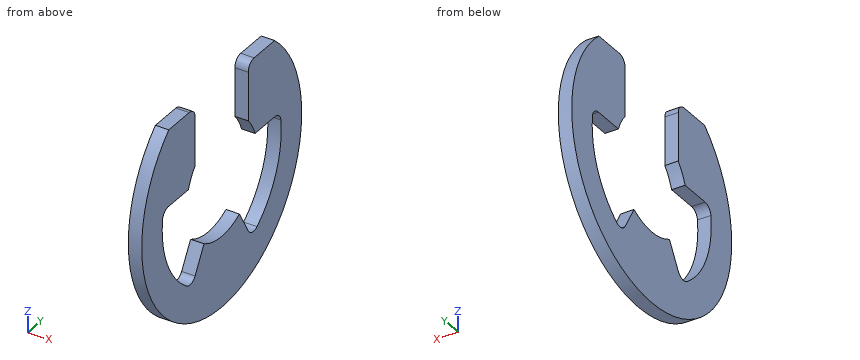
```python
from build123d import *

# Parameters (mm, degrees)
EXTRUDE1_DEPTH = 0.4445
FILLET1_R      = 0.6223


with BuildPart() as part:
    # Sketch1 → Extrude1 (new body, symmetric)
    with BuildSketch(Plane(origin=(0, 0, 0), x_dir=(0, 0, -1), z_dir=(1, 0, 0))):
        with BuildLine():
            Line((-2.45287604, 2.7813), (-6.2865, 2.7813))
            Line((-6.2865, 2.7813), (-6.2865, 5.544171872))
            ThreePointArc((-6.2865, 5.544171872), (8.382, 0), (-6.2865, -5.544171872))
            Line((-6.2865, -5.544171872), (-6.2865, -2.7813))
            Line((-6.2865, -2.7813), (-2.45287604, -2.7813))
            ThreePointArc((-2.45287604, -2.7813), (-1.878831673, -3.197220997), (-1.236133333, -3.49631305))
            Line((-1.236133333, -3.49631305), (-1.236133333, -6.116547306))
            ThreePointArc((-1.236133333, -6.116547306), (2.566674294, -5.687913469), (5.404177312, -3.120103226))
            Line((5.404177312, -3.120103226), (3.211568607, -1.8542))
            ThreePointArc((3.211568607, -1.8542), (3.7084, 0), (3.211568607, 1.8542))
            Line((3.211568607, 1.8542), (5.404177312, 3.120103226))
            ThreePointArc((5.404177312, 3.120103226), (2.566674294, 5.687913469), (-1.236133333, 6.116547306))
            Line((-1.236133333, 6.116547306), (-1.236133333, 3.49631305))
            ThreePointArc((-1.236133333, 3.49631305), (-1.878831673, 3.197220997), (-2.45287604, 2.7813))
        make_face()
    extrude(amount=EXTRUDE1_DEPTH, both=True)

    # Fillet1
    fillet1_edges = [part.edges().sort_by_distance(p)[0] for p in [
        (0, -2.7813, 6.2865),
        (0, -6.116547306, 1.236133333),
        (0, -3.120103226, -5.404177312),
        (0, 3.120103226, -5.404177312),
        (0, 6.116547306, 1.236133333),
        (0, 2.7813, 6.2865),
    ]]
    fillet(fillet1_edges, radius=FILLET1_R)


solid = part.part
```
Geometry check sheet. Reference: the model listing, model coordinates, mm. Give positions to 0.01 mm unless a question says otherwise; leave off trailing zeros. Write each loop counter-clockwise with the first axis right and the second up, starting at its lowest first coordinate (ties: lowest second). Pieces come first, ordered by that corner, then holes.
1) Section check C-C, the plane z = -3.5. Record the boundary of the cut face in (x, y).
2) Section check D-D, the plane y = 0. Record the boundary of the cut face in (x, z), and give its area (3 significant figures).
3) Section check B-B, the plane x = -0.3. Record the boundary of the cut face in (y, z).
4) Section check A-A, the plane z = 0. Record the boundary of the cut face in (x, y).
5) Material ranges on L1, parallel to Y at x = -0.1, z = -4; L2, parallel to Y at x = -0.2, z = -4.25; L3, parallel to Y at x = 0.35, z = -3, recorded low to high.
Computed:
1. outline: (-0.44, -7.62) - (0.44, -7.62) - (0.44, -5.17) - (-0.44, -5.17) - close; (-0.44, -2.02) - (0.44, -2.02) - (0.44, -1.23) - (-0.44, -1.23) - close; (-0.44, 1.23) - (0.44, 1.23) - (0.44, 2.02) - (-0.44, 2.02) - close; (-0.44, 5.17) - (0.44, 5.17) - (0.44, 7.62) - (-0.44, 7.62) - close
2. outline: (-0.44, -8.38) - (0.44, -8.38) - (0.44, -3.71) - (-0.44, -3.71) - close
2. area: 4.15 mm2
3. outline: (-6.2, 0.68) arc R0.62 cw to (-5.58, 1.24) - (-3.5, 1.24) arc R3.71 cw to (-2.78, 2.45) - (-2.78, 5.66) arc R0.62 ccw to (-3.4, 6.29) - (-5.54, 6.29) arc R8.38 ccw (long way) to (5.54, 6.29) - (3.4, 6.29) arc R0.62 ccw to (2.78, 5.66) - (2.78, 2.45) arc R3.71 cw to (3.5, 1.24) - (5.58, 1.24) arc R0.62 cw to (6.2, 0.68) arc R6.24 cw to (3.7, -5.03) arc R0.62 cw to (2.79, -4.84) - (1.85, -3.21) arc R3.71 cw to (-1.85, -3.21) - (-2.79, -4.84) arc R0.62 cw to (-3.7, -5.03) arc R6.24 cw to start
4. outline: (-0.44, -8.38) - (0.44, -8.38) - (0.44, -6.24) - (-0.44, -6.24) - close; (-0.44, 6.24) - (0.44, 6.24) - (0.44, 8.38) - (-0.44, 8.38) - close
5. L1: y = -7.37 to -4.79, -2.31 to 2.31, 4.79 to 7.37
5. L2: y = -7.22 to -4.57, -2.45 to 2.45, 4.57 to 7.22
5. L3: y = -7.83 to -5.47, 5.47 to 7.83
